```python
from build123d import *

# Parameters (mm, degrees)
F2_R            = 5
F3_DEPTH        = 4
F2_W            = 30
F2_H            = 40
F4_DEPTH        = 7.7
F5_D            = 5.4
F9_D            = 3.2
F9_CSINK_D      = 6
F9_CSINK_ANGLE  = 90
F11_D           = 2.9
F11_CSINK_D     = 3.5
F11_CSINK_ANGLE = 50
F12_W           = 22.961332947
F12_H           = 13.7697942555
F13_DEPTH       = 12.1


with BuildPart() as f3:
    # F2 (on Right) → F3 (new body)
    with BuildSketch(Plane.YZ):
        Polygon((-62.1075481176, 10.1446546614), (-19.6075481176, 10.1446546614), (-19.6075481176, 50.1446546614), (-30.1075481176, 50.1446546614), (-45.3845150769, 60.1446546614), (-62.1075481176, 60.1446546614), (-62.1075481176, 50.1446546614), align=None)
        with Locations((-36.1075481176, 34.4446546614)):
            Circle(F2_R, mode=Mode.SUBTRACT)
        with Locations((-51.1075481176, 50.1446546614)):
            Circle(F2_R, mode=Mode.SUBTRACT)
        with Locations((-51.1075481176, 50.1446546614)):
            Circle(F2_R)
        with Locations((-36.1075481176, 34.4446546614)):
            Circle(F2_R)
    extrude(amount=-F3_DEPTH)

    # F2 (on Right) → F4 (join)
    with BuildSketch(Plane.YZ):
        with Locations((-4.6075481176, 30.1446546614)):
            Rectangle(F2_W, F2_H)
        Polygon((-62.1075481176, 10.1446546614), (-19.6075481176, 10.1446546614), (-19.6075481176, 50.1446546614), (-30.1075481176, 50.1446546614), (-45.3845150769, 60.1446546614), (-62.1075481176, 60.1446546614), (-62.1075481176, 50.1446546614), align=None)
        with Locations((-36.1075481176, 34.4446546614)):
            Circle(F2_R, mode=Mode.SUBTRACT)
        with Locations((-51.1075481176, 50.1446546614)):
            Circle(F2_R, mode=Mode.SUBTRACT)
    extrude(amount=F4_DEPTH)

    # F5 (through all)
    with Locations(Plane(origin=(0, 0, 0), x_dir=(0, 1, 0), z_dir=(-1, 0, 0))):
        with Locations((0.3924518824, -40.1446546614), (0.3924518824, -20.1446546614), (-14.6075481176, -20.1446546614)):
            Hole(F5_D / 2)


with BuildPart() as f8_1:
    # F8: instance of F3
    add(f3.part.mirror(Plane.YZ.offset(-10.05)))

    # F11 (through all)
    with Locations(Plane.YZ.offset(-16.1)):
        with Locations((-36.1075481176, 34.4446546614), (-51.1075481176, 50.1446546614)):
            CounterSinkHole(F11_D / 2, F11_CSINK_D / 2, counter_sink_angle=F11_CSINK_ANGLE)


with BuildPart() as f3_1:
    add(f3.part)

    # F9 (through all)
    with Locations(Plane.YZ):
        with Locations((-51.1075481176, 50.1446546614), (-36.1075481176, 34.4446546614)):
            CounterSinkHole(F9_D / 2, F9_CSINK_D / 2, counter_sink_angle=F9_CSINK_ANGLE)

    add(f8_1.part)  # F13 merges F8_1
    # F12 (on face) → F13 (join, through all)
    with BuildSketch(Plane(origin=(-4, 0, 0), x_dir=(0, -1, 0), z_dir=(-1, 0, 0))):
        Polygon((62.1075481176, 10.1446546614), (62.1075481176, 45.4412288964), (42.5688810647, 23.9144489169), (42.5688810647, 10.1446546614), align=None)
        with Locations((31.0882145911, 17.0295517892)):
            Rectangle(F12_W, F12_H)
        Polygon((19.6075481176, 50.1446546614), (19.6075481176, 31.1306696385), (34.7832851112, 50.1446546614), (30.1075481176, 50.1446546614), align=None)
    extrude(amount=F13_DEPTH)


solid = f3_1.part
```
Input: part model. Units: mm. Frame: model coordinates. A direction names the side the tool comes from. Coordinates: 2 decimals unless noted, no trailing zeros. Loops run counter-clockwise (first coordinate to the right, second up) from the corner with the lowest first, then second, coordinate; pieces in that order, holes last. Notation, with made-up numbers: M 63,-23.5 L 101,-23.5 A25 cw 101,0.5 Z; hole C -5,-33 d7. An arc over 180 degrees is marked long. Answer in a Markdown table with one row per item.
1. Section D-D, the plane y = -21. Output: boundary loops of the cut face in (x, z).
Response:
| item | result |
|---|---|
| outline | M -27.8,10.14 L 7.7,10.14 L 7.7,50.14 L -27.8,50.14 Z; hole M -16.1,23.91 L -4,23.91 L -4,32.88 L -16.1,32.88 Z |
2. First-contact query: pin 1 (5 mm diameter, centred on y = 0.39, z = 40.14, fed in from -X); pin 2 (8 mm diameter, centred on x = -16.5, y = -12, fed in from +Z); pin 3 (5 mm diameter, centred on y = -38, z = 36, fed in from -X); pin 4 (3 mm diameter, centred on y = -38.5, z = 34.5, fed in from +X). Flat tips, straight axial feed; report the tip coordinate or a pass-through.
Response:
| item | result |
|---|---|
| pin 1 | passes through |
| pin 2 | stops at z = 50.14 |
| pin 3 | stops at x = -20.1 |
| pin 4 | stops at x = 0 |
3. Draft query along X for faces 1 (the flat face through (7.7, -26, 30)), 2 (the flat face through (-10, -19.608, 34)), 3 (the flat face through (-16.1, -41, 42)), 4 (the cylindrical face through (-18.45, -52.49, 50.58)). Return one class per face: pulls with the +X half, pulls with the -X half, needs draft (parallel to the pull), parting line crosses it, or undercut.
Response:
| item | result |
|---|---|
| face 1 | pulls with the +X half |
| face 2 | undercut |
| face 3 | undercut |
| face 4 | needs draft |
4. Section B-B, the plane y = -9. Output: boundary loops of the cut face in (x, z), then the cut area to 3 significant figures.
Response:
| item | result |
|---|---|
| outline | M -27.8,10.14 L -20.1,10.14 L -20.1,50.14 L -27.8,50.14 Z; M 0,10.14 L 7.7,10.14 L 7.7,50.14 L 0,50.14 Z |
| area | 616 mm2 |
5. Section C-C, the plane z = 15. Output: boundary loops of the cut face in (x, y), then the cut area to 3 significant figures.
Response:
| item | result |
|---|---|
| outline | M -27.8,-62.11 L 7.7,-62.11 L 7.7,10.39 L 0,10.39 L 0,-19.61 L -20.1,-19.61 L -20.1,10.39 L -27.8,10.39 Z |
| area | 1,970 mm2 |
6. Section A-A, the plane x = -10.5. Output: boundary loops of the cut face in (y, z), then the cut area to 3 significant figures.
Response:
| item | result |
|---|---|
| outline | M -62.11,10.14 L -19.61,10.14 L -19.61,23.91 L -42.57,23.91 L -62.11,45.44 Z; M -34.78,50.14 L -19.61,31.13 L -19.61,50.14 Z |
| area | 940 mm2 |
7. Material intervals for line 1 (X direction, y = -44.5, z = 56.5); line 2 (X direction, y = -6.5, z = 30); line 3 (Y direction, x = -23, z = 34), sorted ascending.
Response:
| item | result |
|---|---|
| line 1 | x = -27.8 to -16.1, -4 to 7.7 |
| line 2 | x = -27.8 to -20.1, 0 to 7.7 |
| line 3 | y = -62.11 to -41.09, -31.13 to 10.39 |
8. Reachability of faces 5 (the flat face through (0, -5, 30)), 6 (the cylindrical face through (-2.72, -34.93, 35.53)), 7 (the flat face through (-20.1, -52.3, 51.3)), 8 (the flat face through (-9.965, -27.089, 40.505)), 9 (the flat face through (4, 10.392, 30)) from +Z, -Z, +X, -X, +Y, -Y: full face, straight path, thin tool, end or side. Return the list, or none.
Response:
| item | result |
|---|---|
| face 5 | +Z, -Z, +Y |
| face 6 | +X |
| face 7 | -X |
| face 8 | none |
| face 9 | +Z, -Z, +X, -X, +Y |
